Could you check a few things on this drawing? It's one solid part, dimensions in mm from its lowest x, y, z. Give positions to 0.01 mm unless a question says otherwise; leave off trailing zeros. Loops run counter-clockwise (first coordinate to the right, second up) from the corner with the lowest first, then second, coordinate; pieces in that order, holes last. Notation, with made-up numbers: (88.5, 62.5) - (126.5, 62.5) arc R34 cw to (126.5, 98.5) - close; hole circle Ø9 at (47, 86). An arc over 180 degrees is marked (long way). Use a Markdown table: item, result.
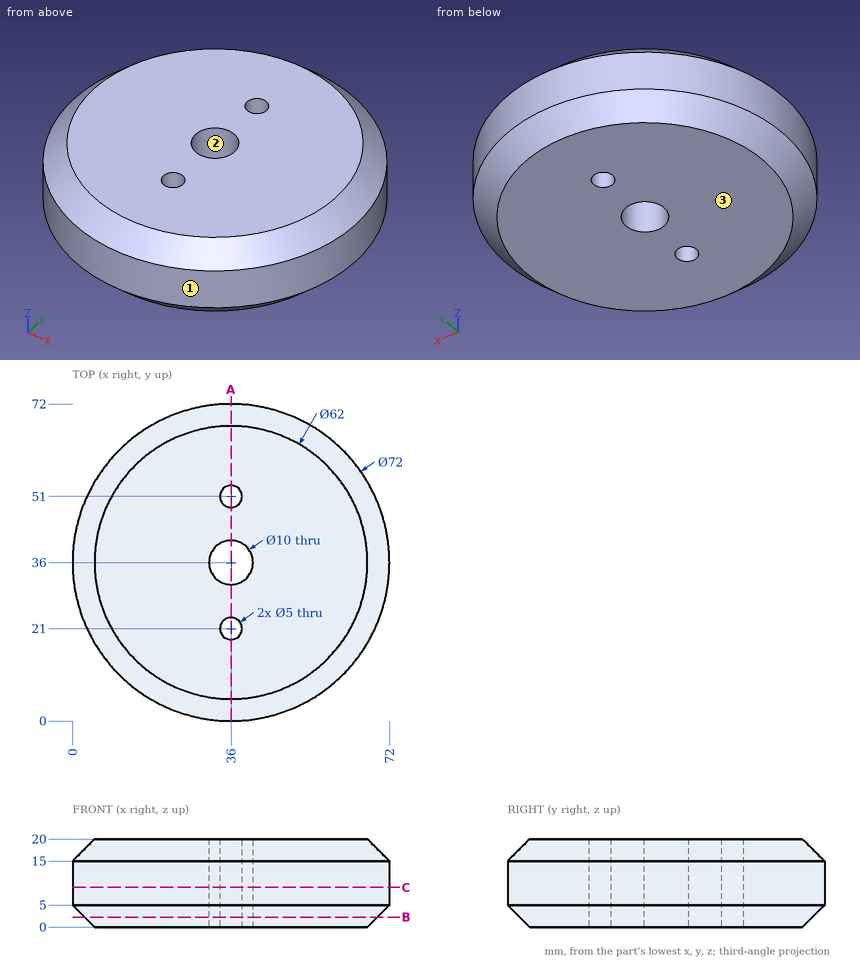
(1) Suppose I cut it at A-A on x = 36. Write out the boundary of the cut face in (y, z).
A:
| item | result |
|---|---|
| outline | (0, 5) - (5, 0) - (18.5, 0) - (18.5, 20) - (5, 20) - (0, 15) - close; (23.5, 0) - (31, 0) - (31, 20) - (23.5, 20) - close; (41, 0) - (48.5, 0) - (48.5, 20) - (41, 20) - close; (53.5, 0) - (67, 0) - (72, 5) - (72, 15) - (67, 20) - (53.5, 20) - close |
(2) Will these pins go through, and if not, where does the flat tip stop? pin 1 (6 mm diameter, centred on x = 15, z = 17.5, fed in from -Y); pin 2 (1 mm diameter, centred on y = 36.5, z = 2.5, fed in from -X); pin 3 (1 mm diameter, centred on y = 30, z = 4, fed in from +X); pin 4 (3 mm diameter, centred on x = 36, y = 21, fed in from -Z).
A:
| item | result |
|---|---|
| pin 1 | y = 5.64 |
| pin 2 | x = 2 |
| pin 3 | x = 71 |
| pin 4 | through |
(3) Suppose I cut it at C-C on z = 9. Write out the boundary of the cut face in (x, y), plus the area to 3 significant figures.
A:
| item | result |
|---|---|
| outline | circle Ø72 at (36, 36); hole circle Ø10 at (36, 36); hole circle Ø5 at (36, 21); hole circle Ø5 at (36, 51) |
| area | 3,950 mm2 |
(4) If I drill on line 1 (Y direction, x = 36, z = 8.5); line 2 (Y direction, x = 36, z = 15.5); line 3 (X direction, y = 39.5, z = 13.75), over which ranges is the centre line in solid material (lowest first)?
A:
| item | result |
|---|---|
| line 1 | 0 to 18.5, 23.5 to 31, 41 to 48.5, 53.5 to 72 |
| line 2 | 0.5 to 18.5, 23.5 to 31, 41 to 48.5, 53.5 to 71.5 |
| line 3 | 0.17 to 32.43, 39.57 to 71.83 |
(5) Suppose I cut it at B-B on z = 2.25. Write out the boundary of the cut face in (x, y), plus the area to 3 significant figures.
A:
| item | result |
|---|---|
| outline | circle Ø66.5 at (36, 36); hole circle Ø10 at (36, 36); hole circle Ø5 at (36, 21); hole circle Ø5 at (36, 51) |
| area | 3,360 mm2 |
(6) We'd pull the mould along X, two halves only. Please class the marked faces 1, 2 and 3: pulls with the +X half, pulls with the -X half, needs draft (parallel to the pull), parting line crosses it, or undercut.
A:
| item | result |
|---|---|
| face 1 | parting line crosses it |
| face 2 | undercut |
| face 3 | needs draft |
